For this review, take the finished solid that the model builds, in its own axes (mm). A direction names the side the tool comes from. Give positions to 0.01 mm unless a question says otherwise; leave off trailing zeros. Loops run counter-clockwise (first coordinate to the right, second up) from the corner with the lowest first, then second, coordinate; pieces in that order, holes last. Notation, with made-up numbers: (51, 19) - (83, 19) arc R26 ccw to (83, 58) - close; hole circle Ø6 at (-12.5, 70). An arc over 180 degrees is marked (long way). Use CSV: the item, a comma, the result in double quotes. Start each with the question number.
1. Take a section at C-C on y = 8.5. Give the boundary of the cut face in (x, z) (3 decimals).
2. Take a section at B-B on z = -9. Give the boundary of the cut face in (x, y).
3. For faces 4 (the flat face through (-22, -20, 0)), 5 (the flat face through (-1.215, -22, 1)), list the 3-axis set-ups (+Z, -Z, +X, -X, +Y, -Y) from which the entire face can be reached by the end or side of a thin tool; tool diameter is ignored.
4. Mouldability with a two-part tool opening along Z and no side actions: class faces 1 (the cylindrical face through (-33.19, 1.005, 1.565)), 2 (the cylindrical face through (-33.054, -53.824, -8.264)), 3 (the flat face through (-22, -54, -22.225)) as pulls with the +Z half, pulls with the -Z half, needs draft (parallel to the pull), parting line crosses it, or undercut.
5. Take a section at A-A on x = -6.5. Give the boundary of the cut face in (y, z) (3 decimals).
6. For pin 1 (6 mm diameter, centred on x = -28.5, z = -13.5, fed in from +Y); pin 2 (2 mm diameter, centred on x = -24, y = -9, fed in from -Z), all flat-tipped, find the tip position at first contact; note any pin that passes through.
7. Take a section at D-D on x = -34.5. Give the boundary of the cut face in (y, z) (3 decimals).
8. Wall thickness on line 1 (Z direction, x = -40.5, y = 6) (3 decimals); line 2 (Y direction, x = -17.5, z = -1); line 3 (Y direction, x = -11.5, z = 2.25): over which ranges is each line inside the solid? List them lowest first.
```python
from build123d import *

# Parameters (mm, degrees)
F0_W     = 41.275
F0_H     = 82.55
F0_R     = 14.2875
F0_H_2   = 3.175
F1_DEPTH = 3.175
F2_DEPTH = 22.225
F4_D     = 6.7564
F4_DEPTH = 76.2
F4_TIP   = 2.0298273432


with BuildPart() as f1:
    # F0 (on Top) → F1 (new body)
    with BuildSketch(Plane.XY):
        with Locations((-21.8522840129, -10.9388585212)):
            Rectangle(F0_W, F0_H)
        with Locations((-21.8522840129, 9.6986414788)):
            Circle(F0_R, mode=Mode.SUBTRACT)
        with Locations((-21.8522840129, -53.8013585212)):
            Rectangle(F0_W, F0_H_2)
    extrude(amount=F1_DEPTH)

    # F0 (on Top) → F2 (join)
    with BuildSketch(Plane.XY):
        with Locations((-21.8522840129, -53.8013585212)):
            Rectangle(F0_W, F0_H_2)
    extrude(amount=-F2_DEPTH)

    # F4
    with Locations(Plane(origin=(0, -52.2138585212, 0), x_dir=(-1, 0, 0), z_dir=(0, 1, 0))):
        with Locations((8.8347840129, -11.1125), (34.8697840129, -11.1125)):
            Hole(F4_D / 2, depth=F4_DEPTH)
            with Locations((0, 0, -(F4_DEPTH + F4_TIP / 2))):  # 118° drill point
                Cone(0, F4_D / 2, F4_TIP, mode=Mode.SUBTRACT)


solid = f1.part
```
Check result:
1,outline,"(-42.49, 0) - (-36.089, 0) - (-36.089, 3.175) - (-42.49, 3.175) - close; (-7.615, 0) - (-1.215, 0) - (-1.215, 3.175) - (-7.615, 3.175) - close"
2,outline,"(-42.49, -55.39) - (-37.51, -55.39) - (-37.51, -52.21) - (-42.49, -52.21) - close; (-32.23, -55.39) - (-11.47, -55.39) - (-11.47, -52.21) - (-32.23, -52.21) - close; (-6.2, -55.39) - (-1.21, -55.39) - (-1.21, -52.21) - (-6.2, -52.21) - close"
3,face 4,"-Z, +X, -X, +Y"
3,face 5,"+Z, -Z, +X, +Y, -Y"
4,face 1,"needs draft"
4,face 2,"undercut"
4,face 3,"pulls with the -Z half"
5,outline,"(-55.389, -22.225) - (-52.214, -22.225) - (-52.214, -13.554) - (-55.389, -13.554) - close; (-55.389, -8.671) - (-52.214, -8.671) - (-52.214, 0) - (30.336, 0) - (30.336, 3.175) - (-55.389, 3.175) - close"
6,pin 1,"stops at y = -52.21"
6,pin 2,"stops at z = 0"
7,outline,"(-55.389, -22.225) - (-52.214, -22.225) - (-52.214, -14.47) - (-55.389, -14.47) - close; (-55.389, -7.755) - (-52.214, -7.755) - (-52.214, 0) - (3.053, 0) - (3.053, 3.175) - (-55.389, 3.175) - close; (16.345, 0) - (30.336, 0) - (30.336, 3.175) - (16.345, 3.175) - close"
8,line 1,"z = 0 to 3.175"
8,line 2,"y = -55.39 to -52.21"
8,line 3,"y = -55.39 to -0.15, 19.55 to 30.34"
